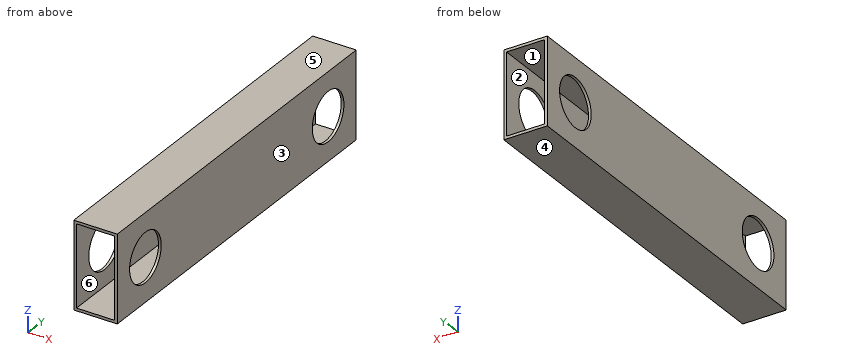
Autodesk Inventor part; units mm, degrees
ref_plane "YZ Plane" through (0, 0, 0) normal (1, 0, 0) x (0, 1, 0)
ref_plane "XZ Plane" through (0, 0, 0) normal (0, 1, 0) x (-1, 0, 0)
ref_plane "XY Plane" through (0, 0, 0) normal (0, 0, 1) x (1, 0, 0)
sketch "Sketch1" plane through (0, 0, 0) normal (0, 1, 0) x (-1, 0, 0)
  line L0 (-12.7, 25.4) -> (12.7, 25.4)
  line L1 (12.7, 25.4) -> (12.7, -25.4)
  line L2 (12.7, -25.4) -> (-12.7, -25.4)
  line L3 (-12.7, -25.4) -> (-12.7, 25.4)
  line L4 (-12.7, 25.4) -> (12.7, -25.4) construction
  line L5 (12.7, 25.4) -> (-12.7, -25.4) construction
  line L6 (11.1125, 23.8125) -> (-11.1125, 23.8125)
  line L7 (-11.1125, 23.8125) -> (-11.1125, -23.8125)
  line L8 (-11.1125, -23.8125) -> (11.1125, -23.8125)
  line L9 (11.1125, -23.8125) -> (11.1125, 23.8125)
  line L10 (11.1125, 23.8125) -> (-11.1125, -23.8125) construction
  line L11 (-11.1125, 23.8125) -> (11.1125, -23.8125) construction
  point P0 (0, 0)
  dimension "d0" = 25.4
  dimension "d1" = 50.8
  dimension "d2" = 22.225
  dimension "d3" = 47.625
extrude "Extrusion1" add sketch "Sketch1" along normal blind 215.9
sketch "Sketch2" plane through (12.7, 0, 25.4) normal (1, 0, 0) x (0, 0, -1)
  line L0 (0, 215.9) -> (50.8, 215.9)
  line L1 (0, 0) -> (0, 215.9)
  point P0 (25.4, 0)
  point P1 (25.4, 190.5)
  dimension "d21" = 25.4
  dimension "d24" = 190.5
hole "Hole1" at (12.7, 190.5, 0) direction (-1, 0, 0) diameter 28.575 end through all
sketch "Sketch3" plane through (12.7, 0, 25.4) normal (1, 0, 0) x (0, 0, -1)
  line L0 (50.8, 0) -> (50.8, 215.9)
  line L1 (0, 0) -> (50.8, 0)
  point P0 (25.4, 0)
  point P1 (25.4, 25.4)
  dimension "d22" = 25.4
  dimension "d23" = 25.4
hole "Hole2" at (12.7, 25.4, 0) direction (-1, 0, 0) diameter 28.575 end through all
properties part number "2x1 Front" material "Aluminum 6061"
Input: part model. Units: mm. Frame: model coordinates. Face numbers are marked on the shaded views. A direction names the side the tool comes from. Coordinates: 2 decimals unless noted, no trailing zeros. Write each loop counter-clockwise with the first axis right and the second up, starting at its lowest first coordinate (ties: lowest second). Pieces come first, ordered by that corner, then holes. Notation, with made-up numbers: (-39, -2) -> (-18, -2) arc R20 cw to (-18, 15) -> close; hole circle Ø2 at (81, 8). An arc over 180 degrees is marked (long way). Write each question's results on one line, items separated by ' | '.
Item 1: Set-up query: the marked faces 5 and 6. Return all of +Z, -Z, +X, -X, +Y, -Y with unobstructed straight access to the full face (end or side cutting, diameter ignored); none if empty.
Conclusion:
face 5: +Z, +X, -X, +Y, -Y | face 6: +Y, -Y
Item 2: Pin query (flat end, axial travel): pin 1 Ø3 at (y, z) = (30, 13.5) entering from +X. Return the tip coordinate at first contact, or that it passes through.
Conclusion:
pin 1: stops at x = 12.7
Item 3: Section query C-C on y = 190.5. Return loops of the section in (x, z).
Conclusion:
outline: (-12.7, -25.4) -> (12.7, -25.4) -> (12.7, -14.29) -> (11.11, -14.29) -> (11.11, -23.81) -> (-11.11, -23.81) -> (-11.11, -14.29) -> (-12.7, -14.29) -> close; (-12.7, 14.29) -> (-11.11, 14.29) -> (-11.11, 23.81) -> (11.11, 23.81) -> (11.11, 14.29) -> (12.7, 14.29) -> (12.7, 25.4) -> (-12.7, 25.4) -> close
Item 4: Section query B-B on x = 6.25. Return loops of the section in (y, z), plus the area to 3 significant figures.
Conclusion:
outline: (0, -25.4) -> (215.9, -25.4) -> (215.9, -23.81) -> (0, -23.81) -> close; (0, 23.81) -> (215.9, 23.81) -> (215.9, 25.4) -> (0, 25.4) -> close | area: 685 mm^2
Item 5: Mould query, pull axis Z, two halves, no side actions, for the marked faces 1, 2, 3 and 4. Classes: +Z half, -Z half, draft (parallel to the pull), parting line (faces both ways), or undercut.
Conclusion:
face 1: undercut | face 2: undercut | face 3: draft | face 4: -Z half
Item 6: Section query D-D on y = 142.5. Return loops of the section in (x, z), plus the area to 3 significant figures.
Conclusion:
outline: (-12.7, -25.4) -> (12.7, -25.4) -> (12.7, 25.4) -> (-12.7, 25.4) -> close; hole (-11.11, -23.81) -> (11.11, -23.81) -> (11.11, 23.81) -> (-11.11, 23.81) -> close | area: 232 mm^2
Item 7: Material intervals for probe 1 along Y at (x, z) = (12.1, 0); probe 2 along X at (y, z) = (23.5, -15); probe 3 along Z at (x, y) = (-12.3, 190.5), sorted ascending.
Conclusion:
probe 1: y = 0 to 11.11, 39.69 to 176.21, 204.79 to 215.9 | probe 2: x = -12.7 to -11.11, 11.11 to 12.7 | probe 3: z = -25.4 to -14.29, 14.29 to 25.4
Item 8: Section query A-A on z = 0. Return loops of the section in (x, y), plus the area to 3 significant figures.
Conclusion:
outline: (-12.7, 0) -> (-11.11, 0) -> (-11.11, 11.11) -> (-12.7, 11.11) -> close; (-12.7, 39.69) -> (-11.11, 39.69) -> (-11.11, 176.21) -> (-12.7, 176.21) -> close; (-12.7, 204.79) -> (-11.11, 204.79) -> (-11.11, 215.9) -> (-12.7, 215.9) -> close; (11.11, 0) -> (12.7, 0) -> (12.7, 11.11) -> (11.11, 11.11) -> close; (11.11, 39.69) -> (12.7, 39.69) -> (12.7, 176.21) -> (11.11, 176.21) -> close; (11.11, 204.79) -> (12.7, 204.79) -> (12.7, 215.9) -> (11.11, 215.9) -> close | area: 504 mm^2
